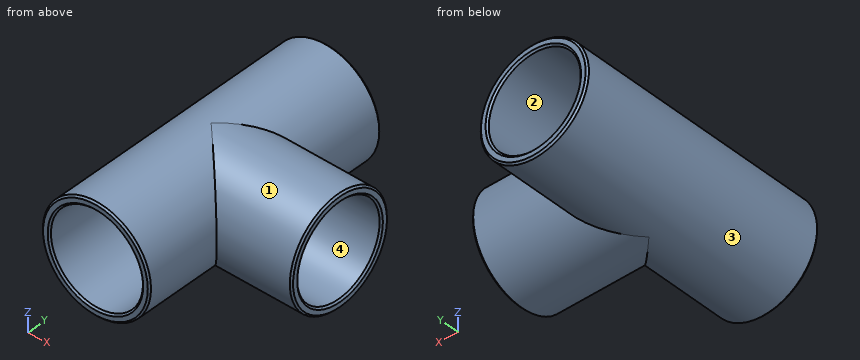
from build123d import *

# Parameters (mm, degrees)
F0_R          = 24.765
F0_R_2        = 21.082
F1_DEPTH      = 59.055
F2_R          = 24.765
F2_R_2        = 21.082
F3_DEPTH      = 59.055
F4_DEPTH      = 59.0560001
F5_DEPTH      = 59.0560001
F5_DEPTH_BACK = 59.0560001
F6_SIZE       = 0.7874
F7_SCALE      = 1.45


with BuildPart() as f1:
    # F0 (on Front) → F1 (new body, symmetric)
    with BuildSketch(Plane.XZ):
        Circle(F0_R)
        Circle(F0_R_2, mode=Mode.SUBTRACT)
    extrude(amount=F1_DEPTH, both=True)

    # F2 (on Right) → F3 (join)
    with BuildSketch(Plane.YZ):
        Circle(F2_R)
        Circle(F2_R_2, mode=Mode.SUBTRACT)
    extrude(amount=F3_DEPTH)

    # F2 (on Right) → F4 (cut, through all)
    with BuildSketch(Plane.YZ):
        Circle(F2_R_2)
    extrude(amount=F4_DEPTH, mode=Mode.SUBTRACT)

    # F0 (on Front) → F5 (cut, two sides)
    with BuildSketch(Plane.XZ) as f5_sk:
        Circle(F0_R_2)
    extrude(amount=F5_DEPTH, mode=Mode.SUBTRACT)
    extrude(f5_sk.sketch, amount=-F5_DEPTH_BACK, mode=Mode.SUBTRACT)

    # F6
    f6_edges = [f1.edges().sort_by_distance(p)[0] for p in [
        (-21.082, -59.055, 0),
        (-24.765, -59.055, 0),
        (59.055, -24.765, 0),
        (59.055, -21.082, 0),
        (-21.082, 59.055, 0),
        (-24.765, 59.055, 0),
    ]]
    chamfer(f6_edges, length=F6_SIZE)


with BuildPart() as f1_1:
    # F7: moved
    add(f1.part.scale(F7_SCALE))


solid = f1_1.part
Work out the finished part from the listing and answer in its coordinate system (mm). Face numbers are marked on the shaded views. A direction names the side the tool comes from. Give positions to 0.01 mm unless a question says otherwise; leave off trailing zeros. Order: outer loops, then holes, each group sorted by start corner. A loop starts at its lowest first (then second) coordinate and runs counter-clockwise, first axis right, second up. Notation, with made-up numbers: (13, 71.25) -> (28, 71.25) arc R15 cw to (28, 75.25) -> close; hole circle Ø3 at (27, -40). An arc over 180 degrees is marked (long way). Answer as a JSON object with one key per item and string values. Group by question number.
1. Section A-A on z = 0 is taken. Determine the outline of the cut face in (x, y).
2. The mould has two halves that part along Z. Classify the marked faces 1 and 2: released by +Z, released by -Z, zero draft, split by the parting line, or undercut.
3. Section C-C on x = 51.5 is taken. Determine the outline of the cut face in (y, z), plus the area to 3 significant figures.
4. Flat-ended cylindrical pins translate along their axes: pin 1 Ø3 at (x, y) = (31, 56.5) entering from -Z; pin 2 Ø2 at (x, y) = (37, -7) entering from -Z; pin 3 Ø10 at (y, z) = (63, -4.5) entering from +X. Find the tip coordinate at first contact, or state that the pin passes through.
5. A tool of negligible diameter and unlimited length cuts with its end or side. For the marked faces 3 and 4, from which of +Z, -Z, +X, -X, +Y, -Y can it reach the whole face along a straight path? Write none if from no direction.
6. Section B-B on y = 0 is taken. Determine the outline of the cut face in (x, z).
7. Consider line 1 along X through (y, z) = (50, -1.5); line 2 along Z through (x, y) = (63.5, -0.5); line 3 along Y through (x, z) = (38, 0). Determine where each line is inside the solid, lowest interval first. Write a range as [from, to].
Result sheet:
{
 "1": {"outline": "(-35.91, -84.49) -> (-34.77, -85.63) -> (-31.71, -85.63) -> (-30.57, -84.49) -> (-30.57, 84.49) -> (-31.71, 85.63) -> (-34.77, 85.63) -> (-35.91, 84.49) -> close; (30.57, -84.49) -> (31.71, -85.63) -> (34.77, -85.63) -> (35.91, -84.49) -> (35.91, -35.91) -> (84.49, -35.91) -> (85.63, -34.77) -> (85.63, -31.71) -> (84.49, -30.57) -> (30.57, -30.57) -> close; (30.57, 30.57) -> (84.49, 30.57) -> (85.63, 31.71) -> (85.63, 34.77) -> (84.49, 35.91) -> (35.91, 35.91) -> (35.91, 84.49) -> (34.77, 85.63) -> (31.71, 85.63) -> (30.57, 84.49) -> close"},
 "2": {"face 1": "split by the parting line", "face 2": "undercut"},
 "3": {"outline": "circle Ø71.82 at (0, 0); hole circle Ø61.14 at (0, 0)", "area": "1,120 mm^2"},
 "4": {"pin 1": "stops at z = -20.47", "pin 2": "stops at z = -35.4", "pin 3": "stops at x = 35.91"},
 "5": {"face 3": "none", "face 4": "+X"},
 "6": {"outline": "(0, -35.91) -> (84.49, -35.91) -> (85.63, -34.77) -> (85.63, -31.71) -> (84.49, -30.57) -> (0, -30.57) arc R30.57 cw to (0, 30.57) -> (84.49, 30.57) -> (85.63, 31.71) -> (85.63, 34.77) -> (84.49, 35.91) -> (0, 35.91) arc R35.91 ccw to start"},
 "7": {"line 1": "x = [-35.88, -30.53], [30.53, 35.88]", "line 2": "z = [-35.91, -30.56], [30.56, 35.91]", "line 3": "y = [-35.91, -30.57], [30.57, 35.91]"}
}
